For this review, use the dimensioned drawing (mm, ordinates from the lowest corner) and the shaded views. Coordinates: 2 decimals unless noted, no trailing zeros. Write each loop counter-clockwise with the first axis right and the second up, starting at its lowest first coordinate (ties: lowest second). Pieces come first, ordered by that corner, then holes. Notation, with made-up numbers: M -36.5,73 L -13.5,73 A22 ccw -13.5,105 Z; hole C 16.25,26 d6. An arc over 180 degrees is marked long. Return JSON: item names as keys, results as strings.
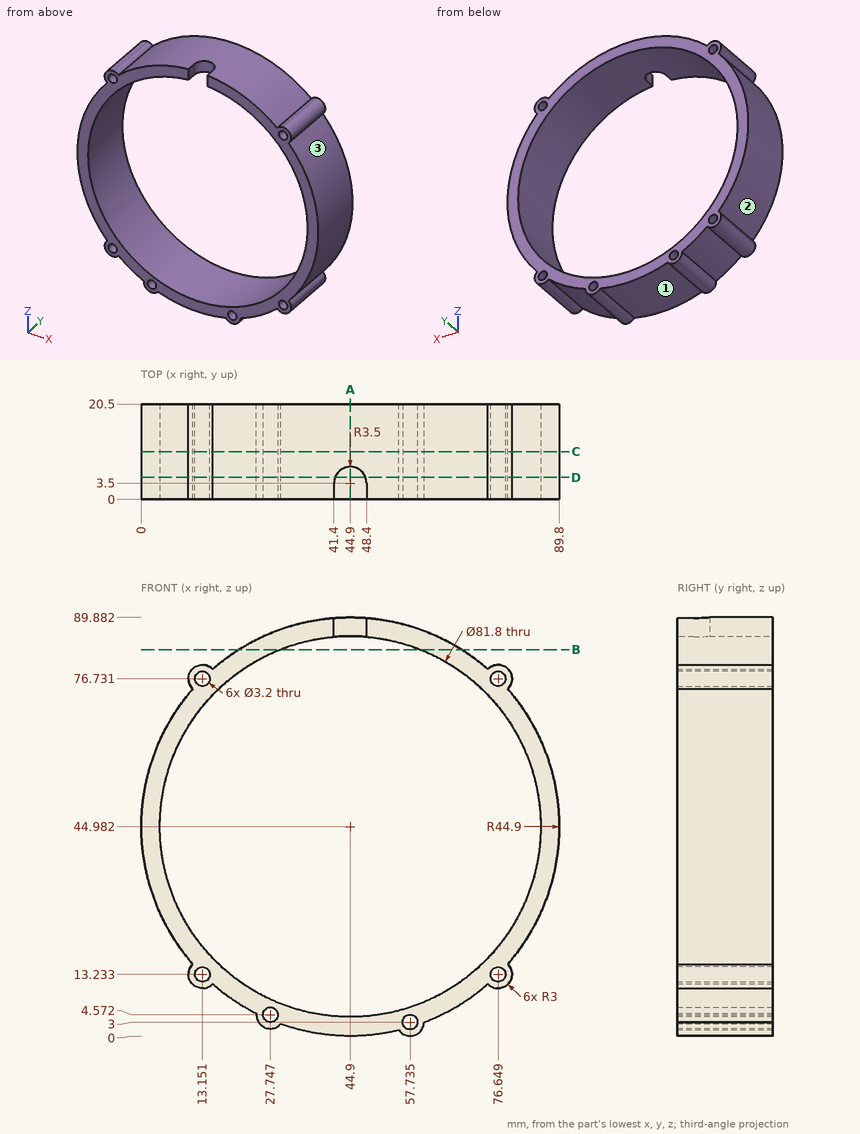
1. Wall thickness on L1, parallel to Z at x = 12, y = 12.5 (1 decimal); L2, parallel to Z at x = 56.5, y = 8.75 (1 decimal); L3, parallel to Z at x = 57.5, y = 4.5: over which ranges is each line inside the solid? List them lowest first. Write a range as from..to.
Checks:
{"L1": "10.5..12.1, 14.3..20.7, 69.3..75.6, 77.8..79.5", "L2": "0.3..2, 4..5.8, 84.2..88.4", "L3": "0.01..1.42, 4.58..6.07, 83.89..88.08"}
2. We need section C-C (y = 10.25). State the section outline as (x, z) points (1 decimal).
Checks:
{"outline": "M 11.1,15.4 A3 ccw long 15.3,11.2 A44.9 ccw 24.8,4.9 A3 ccw 30,2.6 A44.9 ccw 55.3,1.3 A3 ccw 60.7,3 A44.9 ccw 74.5,11.2 A3 ccw long 78.7,15.4 A44.9 ccw 78.7,74.5 A3 ccw long 74.5,78.8 A44.9 ccw 15.3,78.8 A3 ccw long 11.1,74.5 A44.9 ccw Z; hole C 44.9,45 d81.8; hole C 13.2,13.2 d3.2; hole C 13.2,76.7 d3.2; hole C 27.7,4.6 d3.2; hole C 57.7,3 d3.2; hole C 76.6,13.2 d3.2; hole C 76.6,76.7 d3.2"}
3. We need section D-D (y = 4.75). State the section outline as (x, z) points (1 decimal), plus the area to 3 significant figures.
Checks:
{"outline": "M 11.1,15.4 A3 ccw long 15.3,11.2 A44.9 ccw 24.8,4.9 A3 ccw 30,2.6 A44.9 ccw 55.3,1.3 A3 ccw 60.7,3 A44.9 ccw 74.5,11.2 A3 ccw long 78.7,15.4 A44.9 ccw 78.7,74.5 A3 ccw long 74.5,78.8 A44.9 ccw 48.2,89.8 L 48.2,85.8 A40.9 cw long 41.6,85.8 L 41.6,89.8 A44.9 ccw 15.3,78.8 A3 ccw long 11.1,74.5 A44.9 ccw Z; hole C 13.2,13.2 d3.2; hole C 13.2,76.7 d3.2; hole C 27.7,4.6 d3.2; hole C 57.7,3 d3.2; hole C 76.6,13.2 d3.2; hole C 76.6,76.7 d3.2", "area": "1,080 mm2"}
4. We need section B-B (z = 83). State the section outline as (x, y) points.
Checks:
{"outline": "M 21.01,0 L 29.82,0 L 29.82,20.5 L 21.01,20.5 Z; M 59.98,0 L 68.79,0 L 68.79,20.5 L 59.98,20.5 Z"}
5. We need section A-A (x = 44.9). State the section outline as (y, z) points, plus the area to 3 significant figures.
Checks:
{"outline": "M 0,0.08 L 20.5,0.08 L 20.5,4.08 L 0,4.08 Z; M 7,85.88 L 20.5,85.88 L 20.5,89.88 L 7,89.88 Z", "area": "136 mm2"}
6. Draft analysis for pull direction X (two halves, no side actions). For the marked faces 1, 2 and 3, state which applies: +X half, -X half, draft (parallel to the pull), parting line (faces both ways), or undercut.
Checks:
{"face 1": "undercut", "face 2": "-X half", "face 3": "+X half"}
7. Clearance check with flat-ended pins moving along their axes: pin 1 Ø3 at (y, z) = (11.5, 46) entering from -X; pin 2 Ø6 at (y, z) = (14, 54) entering from -X (1 decimal); pin 3 Ø12 at (x, y) = (52.5, 6) entering from +Z; pin 4 Ø1.5 at (x, y) = (50, 18) entering from +Z. State where each tip first meets the part, or that it passes through.
Checks:
{"pin 1": "x = 0", "pin 2": "x = 0.4", "pin 3": "z = 89.85", "pin 4": "z = 89.67"}
